Autodesk Inventor part; units mm, degrees
ref_plane "YZ Plane" through (0, 0, 0) normal (1, 0, 0) x (0, 1, 0)
ref_plane "XZ Plane" through (0, 0, 0) normal (0, 1, 0) x (-1, 0, 0)
ref_plane "XY Plane" through (0, 0, 0) normal (0, 0, 1) x (1, 0, 0)
sketch "草图1" plane through (0, 0, 0) normal (0, 1, 0) x (-1, 0, 0)
  circle A0 centre (0, 0) radius 15
  arc A1 (38.5135, -7.8555) -> (38.5135, 7.8555) centre (37, 0) ccw
  line L0 (38.5135, -7.8555) -> (2.8378, -14.7291)
  line L1 (2.8378, 14.7291) -> (39.6131, 7.6437)
  line L2 (50.7291, 0) -> (-22.1307, 0)
  arc A2 (37, -3.5) -> (37, 3.5) centre (37, 0) ccw
  arc A3 (22, 3.5) -> (22, -3.5) centre (22, 0) ccw
  line L3 (37, -3.5) -> (22, -3.5)
  line L4 (22, 3.5) -> (37, 3.5)
  dimension "d0" = 30
  dimension "d1" = 16
  dimension "d2" = 37
  dimension "d3" = 7
  dimension "d4" = 7
  dimension "d5" = 15
extrude "拉伸1" add sketch "草图1" along normal blind 6 contours L2 A0 | L2 A3 L3 A2 A1 L0 A0 | A0 L1 A1 L2 A2 L4 A3 | A0 L2
sketch "草图2" plane through (0, 6, 0) normal (0, 1, 0) x (1, 0, 0)
  line L0 (-37, 3.5) -> (-22, 3.5)
  arc A0 (-22, -3.5) -> (-22, 3.5) centre (-22, 0) ccw
  line L1 (-22, -3.5) -> (-37, -3.5)
  arc A1 (-37, 3.5) -> (-37, -3.5) centre (-37, 0) ccw
  arc A2 (-38.5135, 7.8555) -> (-38.5135, -7.8555) centre (-37, 0) ccw
  line L2 (-38.5135, -7.8555) -> (-2.8378, -14.7291)
  arc A3 (-2.8378, -14.7291) -> (-2.8378, 14.7291) centre (0, 0) ccw
  line L3 (-2.8378, 14.7291) -> (-38.5135, 7.8555)
  circle A4 centre (0, 0) radius 15
extrude "拉伸2" add sketch "草图2" along normal blind 12 contours A3 A4
sketch "草图3" plane through (0, 18, 0) normal (0, 1, 0) x (1, 0, 0)
  circle A0 centre (0, 0) radius 15
  circle A1 centre (0, 0) radius 9
  dimension "d10" = 18
extrude "拉伸3" cut sketch "草图3" against normal blind 20 contours A1
sketch "草图4" plane through (0, 18, 0) normal (0, 1, 0) x (1, 0, 0)
  circle A0 centre (0, 0) radius 9
  circle A1 centre (0, 0) radius 15
  line L0 (9, 0) -> (15, 0)
  line L1 (6.364, 6.364) -> (10.6066, 10.6066)
  dimension "d13" = 45
extrude "拉伸4" add sketch "草图4" along normal blind 6 contours A0 L1 A1 L0 picked at (12.295, 4.0369)
sketch "草图5" plane through (0, 18, 0) normal (0, 1, 0) x (1, 0, 0)
  arc A0 (10.6066, 10.6066) -> (15, 0) centre (0, 0) ccw
  line L0 (15, 0) -> (9, 0)
  arc A1 (6.364, 6.364) -> (9, 0) centre (0, 0) ccw
  line L1 (0, 0) -> (21.2132, -21.2132) construction
  line L2 (26.5165, -15.9099) -> (14.4889, -3.8823)
  line L3 (3.8823, -14.4889) -> (15.9099, -26.5165)
  line L4 (26.5165, -15.9099) -> (1.7678, -12.3744) construction
  line L5 (12.3744, -1.7678) -> (15.9099, -26.5165) construction
  arc A2 (19.0919, -14.8492) -> (14.8492, -19.0919) centre (16.9706, -16.9706) ccw
  line L6 (14.8492, -19.0919) -> (19.0919, -23.3345)
  line L7 (19.0919, -14.8492) -> (23.3345, -19.0919)
  line L8 (15.9099, -26.5165) -> (19.0919, -23.3345)
  line L9 (23.3345, -19.0919) -> (26.5165, -15.9099)
  point P0 (14.1421, -14.1421)
  dimension "d16" = 45
  dimension "d17" = 15
  dimension "d20" = 6
extrude "拉伸5" add sketch "草图5" against normal blind 6
Check sheet for the modelled part. Datum: model origin and axes. Units: mm. A direction names the side the tool comes from. Round coordinates to 2 decimals unless told otherwise and drop trailing zeros. Order: outer loops, then holes, each group sorted by start corner. A loop starts at its lowest first (then second) coordinate and runs counter-clockwise, first axis right, second up.
(1) Access from +Z, -Z, +X, -X, +Y, -Y to the whole of each face (thin tool, end or side, straight path). Record for faces 5 (the cylindrical face through (-45, 3, 0)), 6 (the flat face through (24.903, 15.042, 17.523)), 7 (the cylindrical face through (13.72, 11.92, -6.06)), 8 (the flat face through (13, 12, 15)), 9 (the flat face through (-30, 3, -3.5)).
(2) Cross-section at D-D, the plane x = -8. Enter the section's corners in (y, z).
(3) Scan lines: probe 1 along X at (y, z) = (7.25, 0); probe 2 along Y at (x, z) = (-28, -7). Record each from-to range of solid material in increasing order.
(4) Cross-section at B-B, the plane x = -24. Enter the section's corners in (y, z).
(5) Cross-section at A-A, the plane z = -2. Enter the section's corners in (x, y), and give its area (3 significant figures).
(6) Go/stop test with flat-tipped pins: P1, Ø11.5, axis at x = 20, z = 17.5, coming from the -Y side; P2, Ø6, axis at x = 2.5, y = 11.5, coming from the -Z side; P3, Ø1, axis at y = 20, z = -2, coming from the +X side; P4, Ø3, axis at x = 13.5, y = 22, coming from the +Z side. Record where each tip stops, or that it passes through.
(7) Draft check along X on faces 1 (the cylindrical face through (-15, 12, 0)), 2 (the flat face through (20.587, 15.042, 9.98)), 3 (the flat face through (12, 21, 0)), 4 (the cylindrical face through (8.584, 9.501, -2.703)). Enter one of: pulls with the +X half, pulls with the -X half, needs draft (parallel to the pull), parting line crosses it, or undercut.
(8) Cross-section at C-C, the plane y = 3. Enter the section's corners in (x, z).
Check sheet entries:
1. face 5: -X, +Y, -Y
1. face 6: +Z, +X, +Y, -Y
1. face 7: -Y
1. face 8: +Z, +X, -Y
1. face 9: +Y, -Y
2. outline: (0, -13.73) - (6, -13.73) - (6, -12.69) - (18, -12.69) - (18, -4.12) - (0, -4.12) - close; (0, 4.12) - (18, 4.12) - (18, 12.69) - (6, 12.69) - (6, 13.73) - (0, 13.73) - close
3. probe 1: x = -15 to -9, 9 to 15
3. probe 2: y = 0 to 6
4. outline: (0, -10.65) - (6, -10.65) - (6, -3.5) - (0, -3.5) - close; (0, 3.5) - (6, 3.5) - (6, 10.65) - (0, 10.65) - close
5. outline: (-44.75, 0) - (-39.87, 0) - (-39.87, 6) - (-44.75, 6) - close; (-19.13, 0) - (-8.77, 0) - (-8.77, 18) - (-14.87, 18) - (-14.87, 6) - (-19.13, 6) - close; (8.77, 0) - (14.87, 0) - (14.87, 6) - (14.87, 24) - (8.77, 24) - close
5. area: 311 mm2
6. P1: stops at y = 12
6. P2: stops at z = -15
6. P3: stops at x = 14.92
6. P4: stops at z = 0
7. face 1: pulls with the -X half
7. face 2: pulls with the +X half
7. face 3: needs draft
7. face 4: undercut
8. outline: (-38.51, -7.86) - (-2.84, -14.73) arc R15 ccw (long way) to (-2.84, 14.73) - (-38.51, 7.86) arc R8 ccw to start; hole (-37, -3.5) - (-22, -3.5) arc R3.5 ccw to (-22, 3.5) - (-37, 3.5) arc R3.5 ccw to start; hole circle Ø18 at (0, 0)
